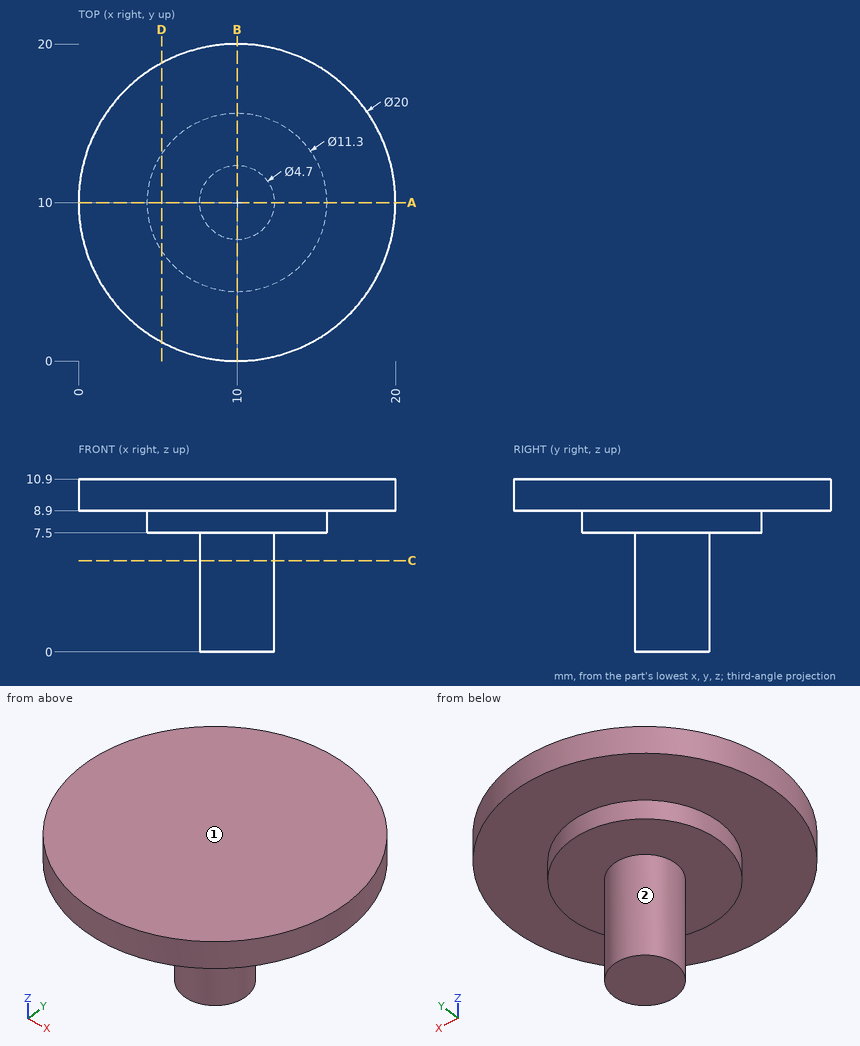
Drawing for the job (mm, zero at the part's lowest x, y, z). A direction names the side the tool comes from. Coordinates: 2 decimals unless noted, no trailing zeros. Loops run counter-clockwise (first coordinate to the right, second up) from the corner with the lowest first, then second, coordinate; pieces in that order, holes last. Notation, with made-up numbers: (18, -23) - (39, -23) arc R15 cw to (39, 4) - close; hole circle Ø5 at (-1.5, -7). An arc over 180 degrees is marked (long way). Return JSON: item names as keys, results as strings.
1. 3-axis set-ups, long thin cutter, end or side, ignore diameter. For the marked faces 1 and 2: which of +Z, -Z, +X, -X, +Y, -Y reach the whole face in a straight line?
Result:
{"face 1": "+Z, +X, -X, +Y, -Y", "face 2": "-Z"}
2. Drop flat-ended pins along their axis: pin 1 (9 mm diameter, centred on x = 8, y = 11.5, fed in from -Z); pin 2 (5 mm diameter, centred on y = 5.5, z = 9.5, fed in from +X); pin 3 (4 mm diameter, centred on x = 18, z = 6, fed in from -Y). Give the stop position or say it passes through.
Result:
{"pin 1": "stops at z = 0", "pin 2": "stops at x = 19.8", "pin 3": "passes through"}
3. Band-saw the part on C-C (z = 5.75). Give the cut face in (x, y).
Result:
{"outline": "circle Ø4.7 at (10, 10)"}
4. Band-saw the part on D-D (x = 5.25). Give the cut face in (y, z), and give its area (3 significant figures).
Result:
{"outline": "(1.2, 8.9) - (6.94, 8.9) - (6.94, 7.5) - (13.06, 7.5) - (13.06, 8.9) - (18.8, 8.9) - (18.8, 10.9) - (1.2, 10.9) - close", "area": "43.8 mm2"}
5. Probe L1, parallel to Z at x = 17, y = 17; L2, parallel to Z at x = 8.25, y = 14.25; L3, parallel to Y at x = 9.25, z = 8.75. List the from-to ranges inside material, lowest first. Write a range as from..to.
Result:
{"L1": "z = 8.9..10.9", "L2": "z = 7.5..10.9", "L3": "y = 4.4..15.6"}
6. Band-saw the part on A-A (y = 10). Give the cut face in (x, z), and give its area (3 significant figures).
Result:
{"outline": "(0, 8.9) - (4.35, 8.9) - (4.35, 7.5) - (7.65, 7.5) - (7.65, 0) - (12.35, 0) - (12.35, 7.5) - (15.65, 7.5) - (15.65, 8.9) - (20, 8.9) - (20, 10.9) - (0, 10.9) - close", "area": "91.1 mm2"}
